from build123d import *

# Parameters (mm, degrees)
F3_R     = 25.4
F4_DEPTH = 25.4
F6_D     = 25.4
F7_R     = 6.34999
F8_R     = 6.35


# Not quite as in the source:
# - a fillet or chamfer is up to 0.001 mm smaller than in the source, because OpenCascade refuses the exact size
# - the program builds the solid bodies; features that only make, move or delete a surface that nothing else refers to are left out


with BuildPart() as f4:
    # F3 (on Front) → F4 (new body)
    with BuildSketch(Plane.XZ):
        Circle(F3_R)
    extrude(amount=F4_DEPTH)

    # F6 (through all)
    with Locations(Plane.XZ.offset(25.4)):
        with Locations((0, 0)):
            Hole(F6_D / 2)

    # F7 (radius 6.35 in the source; OpenCascade refuses exactly that, so slightly less here)
    f7_edges = [f4.edges().sort_by_distance(p)[0] for p in [
        (-25.4, -25.4, 0),
        (-12.7, -25.4, 0),
    ]]
    fillet(f7_edges, radius=F7_R)

    # F8
    f8_edges = [f4.edges().sort_by_distance(p)[0] for p in [
        (-25.4, 0, 0),
    ]]
    fillet(f8_edges, radius=F8_R)


solid = f4.part
Work out the finished part from the listing and answer in its coordinate system (mm). Give positions to 0.01 mm unless a question says otherwise; leave off trailing zeros. Order: outer loops, then holes, each group sorted by start corner. A loop starts at its lowest first (then second) coordinate and runs counter-clockwise, first axis right, second up. Notation, with made-up numbers: (15.25, 18.5) -> (55.25, 18.5) arc R28 ccw to (55.25, 55.5) -> close; hole circle Ø1 at (85, -23). An arc over 180 degrees is marked (long way). Answer as a JSON object with one key per item and string values. Group by question number.
1. Section C-C on y = -8.75 is taken. Determine the outline of the cut face in (x, z), plus the area to 3 significant figures.
2. Section D-D on y = -22.25 is taken. Determine the outline of the cut face in (x, z).
3. Consider line 1 along Z through (x, y) = (0, -10.25); line 2 along X through (y, z) = (-17, 2.5); line 3 along Z through (x, y) = (-7, -7.25). Determine where each line is inside the solid, lowest interval first. Write a range as [from, to].
4. Flat-ended cylindrical pins translate along their axes: pin 1 Ø1.5 at (x, y) = (4, -11.5) entering from -Z; pin 2 Ø12 at (y, z) = (-12, 1) entering from +X; pin 3 Ø12 at (x, y) = (-7.5, -13) entering from -Z; pin 4 Ø2 at (y, z) = (-5, -19) entering from +X. Find the tip coordinate at first contact, or state that the pin passes through.
5. The mould has two halves that part along X. Classify faces 1 (the cylindrical face through (2.75, -9.39, -12.4)), 2 (the flat face through (12.4, 0, -4)), 3 (the cylindrical face through (-5.506, -12.611, -24.796)): released by +X, released by -X, zero draft, split by the parting line, or undercut.
Result sheet:
{
 "1": {"outline": "circle Ø50.8 at (0, 0); hole circle Ø25.4 at (0, 0)", "area": "1,520 mm^2"},
 "2": {"outline": "circle Ø49.07 at (0, 0); hole circle Ø27.13 at (0, 0)"},
 "3": {"line 1": "z = [-25.4, -12.7], [12.7, 25.4]", "line 2": "x = [-25.28, -12.45], [12.45, 25.28]", "line 3": "z = [-24.42, -10.6], [10.6, 24.42]"},
 "4": {"pin 1": "stops at z = -25.19", "pin 2": "stops at x = 25.4", "pin 3": "stops at z = -25.36", "pin 4": "stops at x = 17.75"},
 "5": {"face 1": "undercut", "face 2": "zero draft", "face 3": "split by the parting line"}
}
